```python
from build123d import *

# Parameters (mm, degrees)
SKETCH1_R           = 2.921
SKETCH1_R_2         = 0.762
BOSS_EXTRUDE1_DEPTH = 2.286


with BuildPart() as part:
    # Sketch1 → Boss-Extrude1 (new body)
    with BuildSketch(Plane(origin=(0, 0, 0), x_dir=(1, 0, 0), z_dir=(0, 1, 0))):
        with BuildLine():
            Line((-4.2926, 4.274545315), (-2.466531309, 16.914204067))
            ThreePointArc((-2.466531309, 16.914204067), (0, 19.05), (2.466531309, 16.914204067))
            Line((2.466531309, 16.914204067), (4.2926, 4.274545315))
            ThreePointArc((4.2926, 4.274545315), (6.0579, 0), (4.2926, -4.274545315))
            Line((4.2926, -4.274545315), (2.466531309, -16.914204067))
            ThreePointArc((2.466531309, -16.914204067), (0, -19.05), (-2.466531309, -16.914204067))
            Line((-2.466531309, -16.914204067), (-4.2926, -4.274545315))
            ThreePointArc((-4.2926, -4.274545315), (-6.0579, 0), (-4.2926, 4.274545315))
        make_face()
        Circle(SKETCH1_R, mode=Mode.SUBTRACT)
        with Locations((0, 16.129)):
            Circle(SKETCH1_R_2, mode=Mode.SUBTRACT)
        with Locations((0, 13.0556)):
            Circle(SKETCH1_R_2, mode=Mode.SUBTRACT)
        with Locations((0, 9.9822)):
            Circle(SKETCH1_R_2, mode=Mode.SUBTRACT)
        with Locations((0, 6.9088)):
            Circle(SKETCH1_R_2, mode=Mode.SUBTRACT)
    extrude(amount=BOSS_EXTRUDE1_DEPTH)


solid = part.part
```
The listing builds one solid part. Answer for the finished solid, in the listing's coordinates (mm). Coordinates: 2 decimals unless noted, no trailing zeros. Loops run counter-clockwise (first coordinate to the right, second up) from the corner with the lowest first, then second, coordinate; pieces in that order, holes last. Notation, with made-up numbers: (44, 46.25) - (51, 46.25) arc R22 cw to (51, 69.25) - close; hole circle Ø2 at (-23, 11.5). An arc over 180 degrees is marked (long way). Write item = value, one per line.
1) Section B-B (x = 0) is taken. Determine the outline of the cut face in (y, z), plus the area to 3 significant figures.
Responses:
outline = (0, -19.05) - (2.29, -19.05) - (2.29, -16.89) - (0, -16.89) - close; (0, -15.37) - (2.29, -15.37) - (2.29, -13.82) - (0, -13.82) - close; (0, -12.29) - (2.29, -12.29) - (2.29, -10.74) - (0, -10.74) - close; (0, -9.22) - (2.29, -9.22) - (2.29, -7.67) - (0, -7.67) - close; (0, -6.15) - (2.29, -6.15) - (2.29, -2.92) - (0, -2.92) - close; (0, 2.92) - (2.29, 2.92) - (2.29, 19.05) - (0, 19.05) - close
area = 59.8 mm^2
2) Section A-A (z = 0) is taken. Determine the outline of the cut face in (x, y).
Responses:
outline = (-6.06, 0) - (-2.92, 0) - (-2.92, 2.29) - (-6.06, 2.29) - close; (2.92, 0) - (6.06, 0) - (6.06, 2.29) - (2.92, 2.29) - close
3) Find the intervals of material crossed by line 1 along Z through (x, y) = (0.5, 2.25); line 2 along X through (y, z) = (0.9, 0); line 3 along X through (y, z) = (1.75, -7), in increasing order.
Responses:
line_1 = -19 to -16.7, -15.55 to -13.63, -12.48 to -10.56, -9.41 to -7.48, -6.33 to -2.88, 2.88 to 19
line_2 = -6.06 to -2.92, 2.92 to 6.06
line_3 = -3.9 to -0.76, 0.76 to 3.9
4) Determine the mould class of faces 1 (the face through (-3.367, 1.127, 10.683)), 2 (the face through (0, 2.286, 4)), 3 (the face through (-0.165, 1.127, -6.165)) for opening direction X: pulls with the +X half, pulls with the -X half, needs draft (parallel to the pull), parting line crosses it, or undercut.
Responses:
face_1 = pulls with the -X half
face_2 = needs draft
face_3 = undercut
5) Section D-D (x = -3.75) is taken. Determine the outline of the cut face in (y, z), plus the area to 3 significant figures.
Responses:
outline = (0, -8.03) - (2.29, -8.03) - (2.29, 8.03) - (0, 8.03) - close
area = 36.7 mm^2
6) Section C-C (y = 0.35) is taken. Determine the outline of the cut face in (x, z), plus the area to 3 significant figures.
Responses:
outline = (-4.29, -4.27) - (-2.47, -16.91) arc R2.49 ccw to (2.47, -16.91) - (4.29, -4.27) arc R6.06 ccw to (4.29, 4.27) - (2.47, 16.91) arc R2.49 ccw to (-2.47, 16.91) - (-4.29, 4.27) arc R6.06 ccw to start; hole circle Ø5.84 at (0, 0); hole circle Ø1.52 at (0, -16.13); hole circle Ø1.52 at (0, -13.06); hole circle Ø1.52 at (0, -9.98); hole circle Ø1.52 at (0, -6.91)
area = 247 mm^2
7) Each of these flat-tipped pins is pushed along its axis until it touches: P1, Ø5.5, axis at x = 0, z = 0, coming from the +Y side; P2, Ø1, axis at y = 1, z = 12, coming from the -X side. Where does it stop, or does it pass through?
Responses:
P1 = through
P2 = -3.25
